Could you check a few things on this model? Use its own coordinates, in mm. Face numbers are marked on the shaded views. Give positions to 0.01 mm unless a question says otherwise; leave off trailing zeros. Write each loop counter-clockwise with the first axis right and the second up, starting at its lowest first coordinate (ties: lowest second). Pieces come first, ordered by that corner, then holes. Notation, with made-up numbers: M -40,7.25 L 5,7.25 A25 cw 5,37.25 Z; hole C 6,-17 d2. An arc over 180 degrees is marked long. One line per item, written item: value.
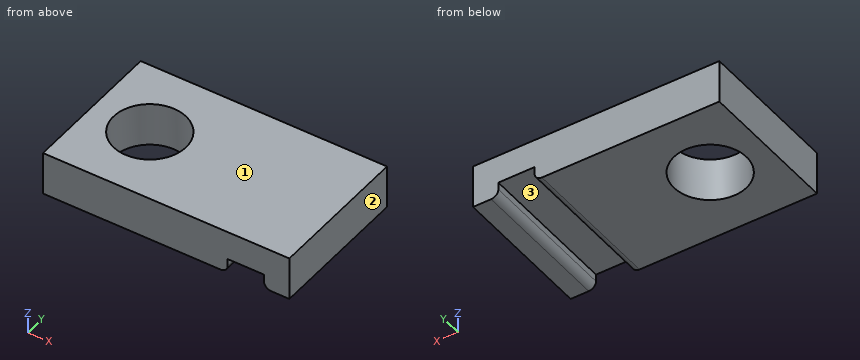
```python
from build123d import *

# Parameters (mm, degrees)
F1_DEPTH      = 5
F1_DEPTH_BACK = 5
F2_R          = 2.5
F3_DEPTH      = 3.001
F4_R          = 0.5


with BuildPart() as f1:
    # F0 (on Front) → F1 (new body, two sides)
    with BuildSketch(Plane.XZ) as f1_sk:
        Polygon((0, 3), (0, 0), (12.75, 0), (12.75, 1), (15.25, 1), (15.25, 0), (17, 0), (17, 3), align=None)
    extrude(amount=F1_DEPTH)
    extrude(f1_sk.sketch, amount=-F1_DEPTH_BACK)

    # F2 (on face) → F3 (cut, through all)
    with BuildSketch(Plane.XY.offset(3)):
        with Locations((4, 0)):
            Circle(F2_R)
    extrude(amount=-F3_DEPTH, mode=Mode.SUBTRACT)

    # F4
    f4_edges = [f1.edges().sort_by_distance(p)[0] for p in [
        (12.75, 0, 0),
        (15.25, 0, 0),
    ]]
    fillet(f4_edges, radius=F4_R)


solid = f1.part
```
1) If we section it at C-C, the plane y = 0: Write out the boundary of the cut face in (x, z).
Outcome:
outline: M 0,0 L 1.5,0 L 1.5,3 L 0,3 Z; M 6.5,0 L 12.25,0 A0.5 ccw 12.75,0.5 L 12.75,1 L 15.25,1 L 15.25,0.5 A0.5 ccw 15.75,0 L 17,0 L 17,3 L 6.5,3 Z
2) If we section it at D-D, the plane x = 4: Write out the boundary of the cut face in (y, z), then the cut area to 3 significant figures.
Outcome:
outline: M -5,0 L -2.5,0 L -2.5,3 L -5,3 Z; M 2.5,0 L 5,0 L 5,3 L 2.5,3 Z
area: 15.0 mm^2
3) Please list where these lines run through material, in increasing order: L1, parallel to Y at x = 4, z = 2.2; L2, parallel to X at y = 1, z = 0.6; L3, parallel to X at y = 0.5, z = 0.55. Write a range as from..to.
Outcome:
L1: y = -5..-2.5, 2.5..5
L2: x = 0..1.71, 6.29..12.75, 15.25..17
L3: x = 0..1.55, 6.45..12.75, 15.25..17
4) If we section it at B-B, the plane x = 6: Write out the boundary of the cut face in (y, z).
Outcome:
outline: M -5,0 L -1.5,0 L -1.5,3 L -5,3 Z; M 1.5,0 L 5,0 L 5,3 L 1.5,3 Z
5) If we section it at A-A, the plane z = 0.2: Write out the boundary of the cut face in (x, y), then the cut area to 3 significant figures.
Outcome:
outline: M 0,-5 L 12.65,-5 L 12.65,5 L 0,5 Z; M 15.35,-5 L 17,-5 L 17,5 L 15.35,5 Z; hole C 4,0 d5
area: 123 mm^2
6) I'm going to push a flat-ended pin straight in: pin 1 (2 mm diameter, centred on x = 14.5, y = 2, fed in from -Z). Where does the tip first touch, or does it pass through?
Outcome:
pin 1: stops at z = 0.07
7) We'd pull the mould along X, two halves only. Please class the marked faces 1, 2 and 3: pulls with the +X half, pulls with the -X half, needs draft (parallel to the pull), parting line crosses it, or undercut.
Outcome:
face 1: needs draft
face 2: pulls with the +X half
face 3: undercut
